Source: CAD feature listing. Evaluate the final solid. Frame: model axes, mm. A direction names the side the tool comes from. Coordinates: 2 decimals unless noted, no trailing zeros. One line per item, written item: value. Start each with the question number.
1. First-contact query: P1, Ø1.5, axis at y = 39.5, z = 18, coming from the +X side; P2, Ø10.5, axis at x = -2, z = 8, coming from the +Y side; P3, Ø19, axis at x = -7, z = -6, coming from the +Y side (3 decimals). Flat tips, straight axial feed; report the tip coordinate or a pass-through.
2. Access query for faces 4 (the flat face through (0, 0, 0)), 5 (the flat face through (-6.02, 51.117, 18.25)), 6 (the cylindrical face through (-13.858, 29.203, 10.626)). Directions: +Z, -Z, +X, -X, +Y, -Y. A direction counts if a zero-diameter tool reaches every point of the face in a straight line with its end or side. Return the directions, or none.
3. Mould query, pull axis X, two halves, no side actions, for faces 1 (the flat face through (6.02, 68.58, 18.25)), 2 (the cylindrical face through (-15.12, 29.05, 11.59)), 3 (the flat face through (0, 6.35, 0)). Classes: released by +X, released by -X, zero draft, split by the parting line, or undercut.
4. Line query: line 1 (Z direction, x = 0, y = 64); line 2 (Z direction, x = 0, y = 21). Output: solid intervals per line, ascending.
from build123d import *

# Parameters (mm, degrees)
SKETCH1_R           = 31.75
BOSS_EXTRUDE1_DEPTH = 6.35


with BuildPart() as part:
    # Sketch1 → Boss-Extrude1 (new body)
    with BuildSketch(Plane(origin=(0, 0, 0), x_dir=(1, 0, 0), z_dir=(0, 1, 0))):
        Circle(SKETCH1_R)
    extrude(amount=BOSS_EXTRUDE1_DEPTH)

    # Sketch2 → Revolve1 (revolve)
    with BuildSketch(Plane.XY):
        Polygon((19.05, 6.35), (19.05, 51.1175), (20.6375, 51.1175), (20.6375, 68.58), (19.05, 68.58), (19.05, 52.705), (17.4625, 52.705), (17.4625, 6.35), align=None)
    revolve(axis=Axis((0, -26.067472827, 0), (0, 1, 0)))


solid = part.part
Computed values:
1. P1: stops at x = 8.08
1. P2: stops at y = 6.35
1. P3: stops at y = 52.705
2. face 4: +Z, -Z, +X, -X, -Y
2. face 5: none
2. face 6: +Y
3. face 1: zero draft
3. face 2: split by the parting line
3. face 3: undercut
4. line 1: z = -20.64 to -19.05, 19.05 to 20.64
4. line 2: z = -19.05 to -17.46, 17.46 to 19.05
